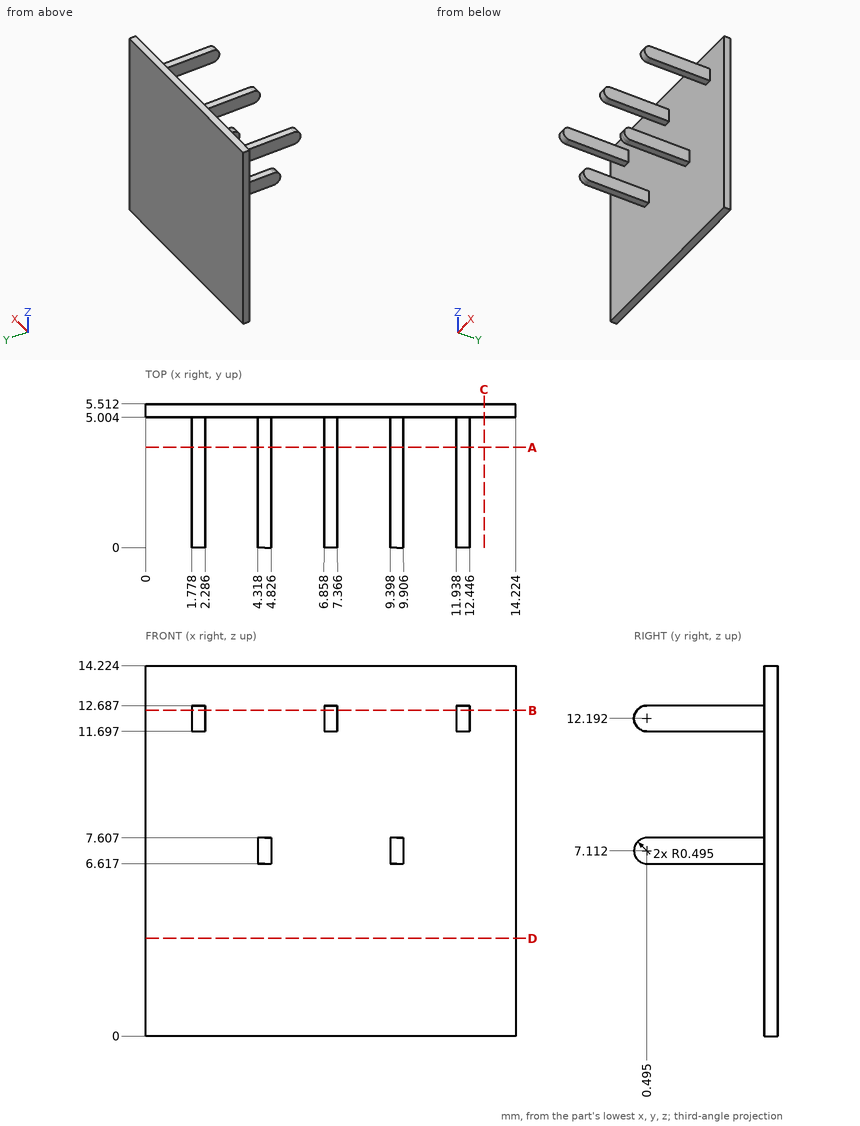
Job drawing, mm, ordinate dimensions from the low corner. One solid piece. Give positions to 0.01 mm unless a question says otherwise; leave off trailing zeros. Write each loop counter-clockwise with the first axis right and the second up, starting at its lowest first coordinate (ties: lowest second). Pieces come first, ordered by that corner, then holes. Notation, with made-up numbers: M 37.25,62.5 L 87.25,62.5 A34 cw 87.25,92.5 Z; hole C -8.5,18.5 d8. An arc over 180 degrees is marked long. Put each result on its own line as item: value. Start each with the question number.
(1) Flat gauge pins, fed straight in: pin 1 Ø1.1 at (y, z) = (3, 7) entering from -X; pin 2 Ø0.5 at (y, z) = (3.5, 12) entering from -X; pin 3 Ø1.1 at (y, z) = (2.5, 12.5) entering from +X. Where does each tip first touch, or does it go through?
(2) Band-saw the part on C-C, the plane x = 13. Write the cut outline in (y, z).
(3) Probe L1, parallel to X at y = 1.8, z = 12; L2, parallel to Y at x = 5.25, z = 10.5; L3, parallel to X at y = 3.9, z = 7. List the from-to ranges inside material, lowest first.
(4) Band-saw the part on A-A, the plane y = 3.85. Write the cut outline in (x, z).
(5) Band-saw the part on D-D, the plane z = 3.75. Write the cut outline in (x, y).
(6) Band-saw the part on B-B, the plane z = 12.5. Write the cut outline in (x, y), and give its area (3 significant figures).
Response values:
1. pin 1: stops at x = 4.32
1. pin 2: stops at x = 1.78
1. pin 3: stops at x = 12.45
2. outline: M 5,0 L 5.51,0 L 5.51,14.22 L 5,14.22 Z
3. L1: x = 1.78 to 2.29, 6.86 to 7.37, 11.94 to 12.45
3. L2: y = 5 to 5.51
3. L3: x = 4.32 to 4.83, 9.4 to 9.91
4. outline: M 1.78,11.7 L 2.29,11.7 L 2.29,12.69 L 1.78,12.69 Z; M 4.32,6.62 L 4.83,6.62 L 4.83,7.61 L 4.32,7.61 Z; M 6.86,11.7 L 7.37,11.7 L 7.37,12.69 L 6.86,12.69 Z; M 9.4,6.62 L 9.91,6.62 L 9.91,7.61 L 9.4,7.61 Z; M 11.94,11.7 L 12.45,11.7 L 12.45,12.69 L 11.94,12.69 Z
5. outline: M 0,5 L 14.22,5 L 14.22,5.51 L 0,5.51 Z
6. outline: M 0,5 L 1.78,5 L 1.78,0.11 L 2.29,0.11 L 2.29,5 L 6.86,5 L 6.86,0.11 L 7.37,0.11 L 7.37,5 L 11.94,5 L 11.94,0.11 L 12.45,0.11 L 12.45,5 L 14.22,5 L 14.22,5.51 L 0,5.51 Z
6. area: 14.7 mm2
